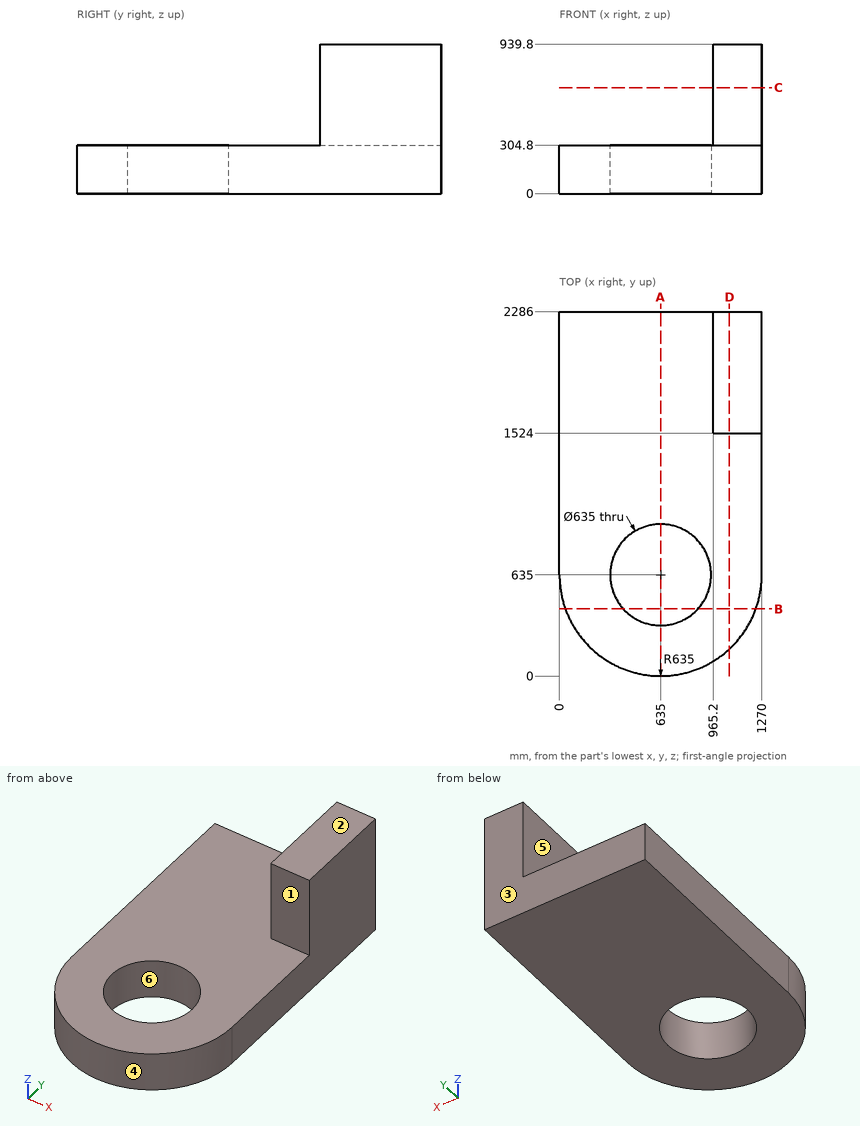
For this review, use the dimensioned drawing (mm, ordinates from the lowest corner) and the shaded views. A direction names the side the tool comes from. Round coordinates to 2 decimals unless told otherwise and drop trailing zeros. Loops run counter-clockwise (first coordinate to the right, second up) from the corner with the lowest first, then second, coordinate; pieces in that order, holes last. Notation, with made-up numbers: M 5.25,-25 L 55.25,-25 A25 cw 55.25,-4 Z; hole C 5,76 d7. An arc over 180 degrees is marked long. Answer as CSV lines item,"result".
1. Insertion check: pin 1 Ø12 at (x, z) = (954, 688) entering from +Y; pin 2 Ø1 at (x, y) = (892.5, 1241.5) entering from +Z. Each pin has a flat end and moves straight along its axis. Give the tip position at first contact, or say it passes through.
Outcome:
pin 1,"passes through"
pin 2,"stops at z = 304.8"
2. We need section C-C (z = 666.5). Give the boundary of the cut face in (x, y), plus the area to 3 significant figures.
Outcome:
outline,"M 965.2,1524 L 1270,1524 L 1270,2286 L 965.2,2286 Z"
area,"232,000 mm2"
3. For the marked faces 1 and 2, list the 3-axis set-ups (+Z, -Z, +X, -X, +Y, -Y) from which the entire face can be reached by the end or side of a thin tool; tool diameter is ignored.
Outcome:
face 1,"+Z, +X, -X, -Y"
face 2,"+Z, +X, -X, +Y, -Y"
4. We need section B-B (y = 422). Give the boundary of the cut face in (x, z).
Outcome:
outline,"M 36.79,0 L 399.55,0 L 399.55,304.8 L 36.79,304.8 Z; M 870.45,0 L 1233.21,0 L 1233.21,304.8 L 870.45,304.8 Z"
5. Draft analysis for pull direction X (two halves, no side actions). For the marked faces 3, 4, 5 and 6, state which applies: pulls with the +X half, pulls with the -X half, needs draft (parallel to the pull), parting line crosses it, or undercut.
Outcome:
face 3,"needs draft"
face 4,"parting line crosses it"
face 5,"pulls with the -X half"
face 6,"undercut"
6. To check wall thickness, follow L1, parallel to Y at x = 651, z = 55; L2, parallel to Y at x = 635, z = 216.5; L3, parallel to Z at x = 413.5, y = 1711. State the ranges of each line that lie inside material, in increasing order. Write a range as [from, to].
Outcome:
L1,"y = [0.2, 317.9], [952.1, 2286]"
L2,"y = [0, 317.5], [952.5, 2286]"
L3,"z = [0, 304.8]"
7. We need section A-A (x = 635). Give the boundary of the cut face in (y, z).
Outcome:
outline,"M 0,0 L 317.5,0 L 317.5,304.8 L 0,304.8 Z; M 952.5,0 L 2286,0 L 2286,304.8 L 952.5,304.8 Z"
8. We need section D-D (x = 1066.5). Give the boundary of the cut face in (y, z), plus the area to 3 significant figures.
Outcome:
outline,"M 169.13,0 L 2286,0 L 2286,939.8 L 1524,939.8 L 1524,304.8 L 169.13,304.8 Z"
area,"1,130,000 mm2"
